Part model, mm, in its own coordinate system. A direction names the side the tool comes from. Give positions to 0.01 mm unless a question says otherwise; leave off trailing zeros. Loops run counter-clockwise (first coordinate to the right, second up) from the corner with the lowest first, then second, coordinate; pieces in that order, holes last. Notation, with made-up numbers: M 57.5,58.5 L 91.5,58.5 A10 cw 91.5,66.5 Z; hole C -4,16.5 d11. An arc over 180 degrees is marked long. Answer in a Markdown table with one row per item.
from build123d import *

# Parameters (mm, degrees)
SKETCH2_R          = 4
CUT_EXTRUDE1_DEPTH = 10


with BuildPart() as part:
    # Sketch1 → Revolve1 (revolve)
    with BuildSketch(Plane(origin=(0, 0, 0), x_dir=(0, 0, -1), z_dir=(1, 0, 0)), mode=Mode.PRIVATE) as revolve1_sk:
        Polygon((30, 45.055178728), (-30, 45.055178728), (-66.2, 63.5), (-76.2, 63.5), (-76.2, 60.5), (-66.2, 60.5), (-30, 42.055178728), (-1.5, 42.055178728), (-1.5, 10), (1.5, 10), (1.5, 42.055178728), (30, 42.055178728), (66.2, 60.5), (76.2, 60.5), (76.2, 63.5), (66.2, 63.5), align=None)
    revolve(revolve1_sk.sketch.rotate(Axis((0, 0, 361.478930537), (0, 0, -1)), 90), axis=Axis((0, 0, 361.478930537), (0, 0, -1)))

    # Sketch2 → Cut-Extrude1 (cut)
    with BuildSketch(Plane(origin=(0, 0, -1.5), x_dir=(-1, 0, 0), z_dir=(0, 0, -1))):
        with Locations((0, 30)):
            Circle(SKETCH2_R)
        with Locations((30, 0)):
            Circle(SKETCH2_R)
        with Locations((0, -30)):
            Circle(SKETCH2_R)
        with Locations((-30, 0)):
            Circle(SKETCH2_R)
    extrude(amount=-CUT_EXTRUDE1_DEPTH, mode=Mode.SUBTRACT)

    # Sketch3 → Revolve2 (revolve)
    with BuildSketch(Plane(origin=(0, 0, 0), x_dir=(0, 0, -1), z_dir=(1, 0, 0)), mode=Mode.PRIVATE) as revolve2_sk:
        with BuildLine():
            Line((-66.2, 139.7), (66.2, 139.7))
            ThreePointArc((66.2, 139.7), (73.271067812, 136.771067812), (76.2, 129.7))
            Line((76.2, 129.7), (76.2, 63.5))
            Line((76.2, 63.5), (66.2, 63.5))
            Line((66.2, 63.5), (30, 45.055178728))
            Line((30, 45.055178728), (-30, 45.055178728))
            Line((-30, 45.055178728), (-66.2, 63.5))
            Line((-66.2, 63.5), (-76.2, 63.5))
            Line((-76.2, 63.5), (-76.2, 129.7))
            ThreePointArc((-76.2, 129.7), (-73.271067812, 136.771067812), (-66.2, 139.7))
        make_face()
        with BuildLine():
            Line((-66.2, 129.7), (66.2, 129.7))
            ThreePointArc((66.2, 129.7), (67.967766953, 128.967766953), (68.7, 127.2))
            Line((68.7, 127.2), (68.7, 71))
            Line((68.7, 71), (63.893575647, 71))
            Line((63.893575647, 71), (27.946787823, 52.684196776))
            Line((27.946787823, 52.684196776), (-28.453212177, 52.684196776))
            Line((-28.453212177, 52.684196776), (-64.4, 71))
            Line((-64.4, 71), (-68.7, 71))
            Line((-68.7, 71), (-68.7, 127.2))
            ThreePointArc((-68.7, 127.2), (-67.967766953, 128.967766953), (-66.2, 129.7))
        make_face(mode=Mode.SUBTRACT)
    revolve(revolve2_sk.sketch.rotate(Axis((0, 0, 155.803154022), (0, 0, -1)), 90), axis=Axis((0, 0, 155.803154022), (0, 0, -1)))


solid = part.part
(1) Drill centre lines: line 1 along Y through (x, z) = (0, 0.35); line 2 along Z through (x, y) = (-85.5, 57.5); line 3 along Y through (x, z) = (-3.5, 21). Where is each one in solid material? Low to high.
Recorded:
| item | result |
|---|---|
| line 1 | y = -139.7 to -129.7, -52.68 to -34, -26 to -10, 10 to 26, 34 to 52.68, 129.7 to 139.7 |
| line 2 | z = -76.2 to -68.7, 68.7 to 76.2 |
| line 3 | y = -139.66 to -129.65, -52.57 to -41.91, 41.91 to 52.57, 129.65 to 139.66 |
(2) Pin check, flat tips, straight feed: pin 1 Ø1 at (x, z) = (-108, 15.5) entering from -Y; pin 2 Ø12 at (x, z) = (-16, 5) entering from +Y; pin 3 Ø4 at (y, z) = (109.5, 38) entering from -X; pin 4 Ø6.5 at (x, y) = (0, 30) entering from -Z. Stop position of each tip, or through.
Recorded:
| item | result |
|---|---|
| pin 1 | stops at y = -89.22 |
| pin 2 | stops at y = 139.34 |
| pin 3 | stops at x = -89.22 |
| pin 4 | passes through |
(3) Saw through at A-A (x = 0). Give the number of separate pieces and of enclosed holes in the cut face, plus the area to 3 significant figures.
Recorded:
| item | result |
|---|---|
| separate pieces | 4 |
| enclosed holes | 2 |
| area | 8,240 mm^2 |
(4) Which spindle directions (+Z, -Z, +X, -X, +Y, -Y) get a long thin tool onto all of the face, cutting with end or side? Do faces 4 (the face through (56, 27, -76.2)), 5 (the face through (0.521, -26.034, -0.021)), 6 (the face through (-28.116, 126.616, -0.927)), 7 (the face through (-13.12, 59.06, 71.13)), 8 (the face through (-13.12, 59.06, -71.27)). Say none if no direction does.
Recorded:
| item | result |
|---|---|
| face 4 | -Z, +X, -X, +Y, -Y |
| face 5 | +Z, -Z |
| face 6 | none |
| face 7 | +Z |
| face 8 | -Z |
(5) Pull direction Y, two halves, no side cores. Call faces 1 (the face through (-30.28, 136.38, -0.93)), 2 (the face through (-56, 27, 76.2)), 3 (the face through (-9, 9, -1.5)): +Y half, -Y half, draft (parallel to the pull), parting line (faces both ways), or undercut.
Recorded:
| item | result |
|---|---|
| face 1 | parting line |
| face 2 | draft |
| face 3 | undercut |
(6) Saw through at B-B (z = 15). Write the cut outline in (x, y), plus the area to 3 significant figures.
Recorded:
| item | result |
|---|---|
| outline | C 0,0 d279.4; C 0,0 d105.37; hole C 0,0 d259.4; hole C 0,0 d84.11 |
| area | 11,600 mm^2 |
